from build123d import *

# Parameters (mm, degrees)
SKETCH1_R           = 35
SKETCH1_R_2         = 20
BOSS_EXTRUDE6_DEPTH = 75
FILLET1_R           = 30


with BuildPart() as part:
    # Sketch1 → Boss-Extrude6 (new body)
    # profile 1 of 4: a face of its own
    with BuildSketch(Plane(origin=(0, 0, 0), x_dir=(1, 0, 0), z_dir=(0, 1, 0))):
        with BuildLine():
            ThreePointArc((-7.5, -34.186985828), (-15.446901808, -31.406897722), (-22.5, -26.809513237))
            Line((-22.5, -26.809513237), (-22.5, -58.046407186))
            Line((-22.5, -58.046407186), (-7.5, -58.046407186))
            Line((-7.5, -58.046407186), (-7.5, -34.186985828))
        make_face()
    # profile 2 of 4: a face of its own
    with BuildSketch(Plane(origin=(0, 0, 0), x_dir=(1, 0, 0), z_dir=(0, 1, 0))):
        with BuildLine():
            Line((22.5, -58.046407186), (22.5, -26.809513237))
            ThreePointArc((22.5, -26.809513237), (15.446901808, -31.406897722), (7.5, -34.186985828))
            Line((7.5, -34.186985828), (7.5, -58.046407186))
            Line((7.5, -58.046407186), (22.5, -58.046407186))
        make_face()
    # profile 3 of 4: a face of its own
    with BuildSketch(Plane(origin=(0, 0, 0), x_dir=(1, 0, 0), z_dir=(0, 1, 0))):
        Circle(SKETCH1_R)
        with Locations(Location((0, 0, 0), (0, 0, 270))):
            Circle(SKETCH1_R_2, mode=Mode.SUBTRACT)
    # profile 4 of 4: a face of its own
    with BuildSketch(Plane(origin=(0, 0, 0), x_dir=(1, 0, 0), z_dir=(0, 1, 0))):
        with BuildLine():
            ThreePointArc((-55, -7.5), (-62.5, 0), (-55, 7.5))
            Line((-55, 7.5), (-34.186985828, 7.5))
            ThreePointArc((-34.186985828, 7.5), (-32.736987087, 12.381020816), (-30.594117082, 17))
            Line((-30.594117082, 17), (-55, 17))
            ThreePointArc((-55, 17), (-72, 0), (-55, -17))
            Line((-55, -17), (-30.594117082, -17))
            ThreePointArc((-30.594117082, -17), (-32.736987087, -12.381020816), (-34.186985828, -7.5))
            Line((-34.186985828, -7.5), (-55, -7.5))
        make_face()
    extrude(amount=BOSS_EXTRUDE6_DEPTH)

    # Fillet1
    fillet1_edges = [part.edges().sort_by_distance(p)[0] for p in [
        (-15, 0, 58.046407186),
        (-15, 75, 58.046407186),
    ]]
    fillet(fillet1_edges, radius=FILLET1_R)


solid = part.part
The listing builds one solid part. Answer for the finished solid, in the listing's coordinates (mm). A direction names the side the tool comes from. Coordinates: 2 decimals unless noted, no trailing zeros. Loops run counter-clockwise (first coordinate to the right, second up) from the corner with the lowest first, then second, coordinate; pieces in that order, holes last.
1) A tool of negligible diameter and unlimited length cuts with its end or side. For faces 1 (the face through (-62.5, 36.98, 0.16)), 2 (the face through (-7.5, 37, 44)), 3 (the face through (-43, 37, 17)), from which of +Z, -Z, +X, -X, +Y, -Y can it reach the whole face along a straight path? Write none if from no direction.
2) Find section A-A on z = 0. Write down the section's boundary in (x, y), then the cut area to 3 significant figures.
3) Flat-ended cylindrical pins translate along their axes: pin 1 Ø1 at (y, z) = (46.5, 25.5) entering from +X; pin 2 Ø4 at (y, z) = (21.5, -21) entering from +X; pin 3 Ø6 at (x, y) = (9.5, 10) entering from -Z. Find the tip coordinate at first contact, or state that the pin passes through.
4) Find section C-C on y = 40. Write down the section's boundary in (x, z).
5) Find section B-B on x = -51. Write down the section's boundary in (y, z), then the cut area to 4 significant figures.
6) Find section D-D on z = 43. Write down the section's boundary in (x, y), then the cut area to 3 significant figures.
7) Find the intervals of material crossed by L1, parallel to X at y = 47, z = 0; L2, parallel to X at y = 38, z = 45; L3, parallel to Z at x = -54.5, y = 61, in increasing order.
Values:
1. face 1: +Y, -Y
1. face 2: +Z, +Y, -Y
1. face 3: +Z, -X, +Y, -Y
2. outline: (-72, 0) - (-62.5, 0) - (-62.5, 75) - (-72, 75) - close; (-35, 0) - (-20, 0) - (-20, 75) - (-35, 75) - close; (20, 0) - (35, 0) - (35, 75) - (20, 75) - close
2. area: 2,960 mm2
3. pin 1: stops at x = 24.49
3. pin 2: stops at x = 29.39
3. pin 3: stops at z = -34.39
4. outline: (-55, -17) - (-30.59, -17) arc R35 ccw (long way) to (22.5, 26.81) - (22.5, 58.05) - (7.5, 58.05) - (7.5, 34.19) arc R35 ccw to (-7.5, 34.19) - (-7.5, 58.05) - (-22.5, 58.05) - (-22.5, 26.81) arc R35 ccw to (-30.59, 17) - (-55, 17) arc R17 ccw to start; hole (-55, -7.5) - (-34.19, -7.5) arc R35 cw to (-34.19, 7.5) - (-55, 7.5) arc R7.5 ccw to start; hole circle Ø40 at (0, 0)
5. outline: (0, -17) - (75, -17) - (75, -7.5) - (0, -7.5) - close; (0, 7.5) - (75, 7.5) - (75, 17) - (0, 17) - close
5. area: 1,425 mm2
6. outline: (-22.5, 3.99) - (-7.5, 3.99) - (-7.5, 71.01) - (-22.5, 71.01) - close; (7.5, 3.99) - (22.5, 3.99) - (22.5, 71.01) - (7.5, 71.01) - close
6. area: 2,010 mm2
7. L1: x = -72 to -62.5, -35 to -20, 20 to 35
7. L2: x = -22.5 to -7.5, 7.5 to 22.5
7. L3: z = -17 to -7.5, 7.5 to 17
